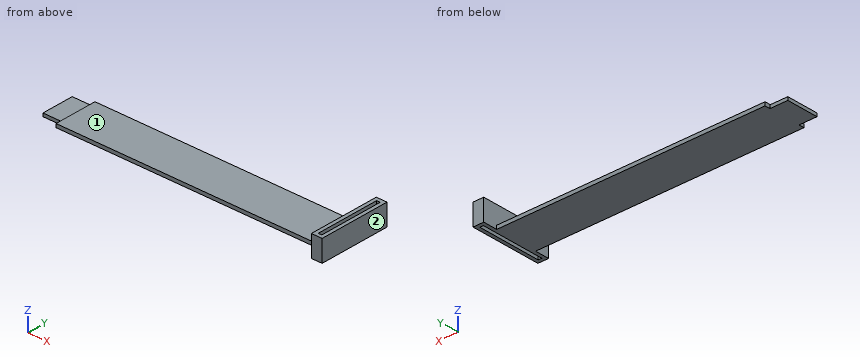
from build123d import *

# Parameters (mm, degrees)
SALIENTE_EXTRUIR1_DEPTH = 2
CROQUIS2_W              = 2
CROQUIS2_H              = 36
SALIENTE_EXTRUIR2_DEPTH = 2
CROQUIS2_2_W            = 2
CROQUIS2_2_H            = 36
SALIENTE_EXTRUIR3_DEPTH = 10
CROQUIS3_W              = 10
CROQUIS3_H              = 1
CORTAR_EXTRUIR1_DEPTH   = 2
CROQUIS4_W              = 10
CROQUIS4_H              = 0.2
CORTAR_EXTRUIR2_DEPTH   = 18


with BuildPart() as part:
    # Croquis1 → Saliente-Extruir1 (new body)
    with BuildSketch(Plane.XY):
        Polygon((-8.516541248, 1.295896328), (1.483458752, 1.295896328), (1.483458752, 3.295896328), (151.483458752, 3.295896328), (151.483458752, -20.704103672), (1.483458752, -20.704103672), (1.483458752, -18.704103672), (-8.516541248, -18.704103672), align=None)
    extrude(amount=SALIENTE_EXTRUIR1_DEPTH)

    # Croquis2 → Saliente-Extruir2 (add)
    with BuildSketch(Plane.XY.offset(2)):
        Polygon((151.483458752, 3.295896328), (151.483458752, 11.295896328), (157.483458752, 11.295896328), (157.483458752, -28.704103672), (151.483458752, -28.704103672), align=None)
        with Locations((154.483458752, -8.704103672)):
            Rectangle(CROQUIS2_W, CROQUIS2_H, mode=Mode.SUBTRACT)
    extrude(amount=-SALIENTE_EXTRUIR2_DEPTH)

    # Croquis2<2> → Saliente-Extruir3 (add)
    with BuildSketch(Plane.XY.offset(2)):
        Polygon((151.483458752, 3.295896328), (151.483458752, 11.295896328), (157.483458752, 11.295896328), (157.483458752, -28.704103672), (151.483458752, -28.704103672), align=None)
        with Locations((154.483458752, -8.704103672)):
            Rectangle(CROQUIS2_2_W, CROQUIS2_2_H, mode=Mode.SUBTRACT)
    extrude(amount=SALIENTE_EXTRUIR3_DEPTH)

    # Croquis3 → Cortar-Extruir1 (cut)
    with BuildSketch(Plane.XY.offset(2)):
        with Locations((-3.516541248, 0.795896328)):
            Rectangle(CROQUIS3_W, CROQUIS3_H)
        with Locations((-3.516541248, -18.204103672)):
            Rectangle(CROQUIS3_W, CROQUIS3_H)
    extrude(amount=-CORTAR_EXTRUIR1_DEPTH, mode=Mode.SUBTRACT)

    # Croquis4 → Cortar-Extruir2 (cut)
    with BuildSketch(Plane.XZ.offset(17.704103672)):
        with Locations((-3.516541248, 1.9)):
            Rectangle(CROQUIS4_W, CROQUIS4_H)
    extrude(amount=-CORTAR_EXTRUIR2_DEPTH, mode=Mode.SUBTRACT)


solid = part.part
Can you work these out from the model? Positions are in its coordinate system, mm. Face numbers are marked on the shaded views. A direction names the side the tool comes from. Round coordinates to 2 decimals unless told otherwise and drop trailing zeros. Write each loop counter-clockwise with the first axis right and the second up, starting at its lowest first coordinate (ties: lowest second). Pieces come first, ordered by that corner, then holes. Notation, with made-up numbers: M 40.5,-15.5 L 54.5,-15.5 A33 ccw 54.5,22.5 Z; hole C 62,-36 d10. An arc over 180 degrees is marked long. Use a Markdown table: item, result.
Item 1: I want a section at A-A (y = 7). List the corners of the cut face in (x, z) for me.
Found:
| item | result |
|---|---|
| outline | M 151.48,0 L 153.48,0 L 153.48,12 L 151.48,12 Z; M 155.48,0 L 157.48,0 L 157.48,12 L 155.48,12 Z |
Item 2: I want a section at D-D (x = 120). List the corners of the cut face in (y, z) for me.
Found:
| item | result |
|---|---|
| outline | M -20.7,0 L 3.3,0 L 3.3,2 L -20.7,2 Z |
Item 3: For pin 1 Ø12 at (x, y) = (112, -4) entering from +Z; pin 2 Ø0.9 at (x, z) = (-1.5, 0.5) entering from +Y; pin 3 Ø3 at (x, y) = (-1.5, -13) entering from +Z, each with a flat end and sliding along its axis, tell me the tip position at first contact or that it passes through.
Found:
| item | result |
|---|---|
| pin 1 | stops at z = 2 |
| pin 2 | stops at y = 0.3 |
| pin 3 | stops at z = 1.8 |
Item 4: If I drill on line 1 along X through (y, z) = (-16, 6.5); line 2 along X through (y, z) = (-6, 1); line 3 along Z through (x, y) = (54.5, 0), over which ranges is the centre line in solid material (lowest first)? Write a range as [from, to].
Found:
| item | result |
|---|---|
| line 1 | x = [151.48, 153.48], [155.48, 157.48] |
| line 2 | x = [-8.52, 153.48], [155.48, 157.48] |
| line 3 | z = [0, 2] |
Item 5: I want a section at C-C (y = -9.5). List the corners of the cut face in (x, z) for me.
Found:
| item | result |
|---|---|
| outline | M -8.52,0 L 153.48,0 L 153.48,12 L 151.48,12 L 151.48,2 L 1.48,2 L 1.48,1.8 L -8.52,1.8 Z; M 155.48,0 L 157.48,0 L 157.48,12 L 155.48,12 Z |
Item 6: Which directions (+Z, -Z, +X, -X, +Y, -Y) give clear straight access to the entire face, cutting with the end or side of a thin tool? Please do the marked faces 1 and 2.
Found:
| item | result |
|---|---|
| face 1 | +Z, -X, +Y, -Y |
| face 2 | +Z, -Z, +X, +Y, -Y |
Item 7: I want a section at B-B (z = 9). List the corners of the cut face in (x, y) for me, and give its area (3 significant figures).
Found:
| item | result |
|---|---|
| outline | M 151.48,-28.7 L 157.48,-28.7 L 157.48,11.3 L 151.48,11.3 Z; hole M 153.48,-26.7 L 155.48,-26.7 L 155.48,9.3 L 153.48,9.3 Z |
| area | 168 mm2 |
